```python
from build123d import *

# Parameters (mm, degrees)
MAINBODYS_W                = 20
MAINBODYS_H                = 28
MAIN_BODY_DEPTH            = 1.6
GROUND_CUT_DEPTH           = 18.278888853
MIDCUTS_W                  = 13
MIDCUTS_H                  = 7
MID_CUT_DEPTH              = 18.278888853
TOPPOWERACCESSCUTS_W       = 11.7
TOPPOWERACCESSCUTS_H       = 6.9
TOP_POWER_ACCESS_CUT_DEPTH = 18.278888853
MC_FILLET_R                = 0.5
ALL_INNER_CUTS_FILLETS_R   = 0.2
OUTER_FILLETS_R            = 1


with BuildPart() as part:
    # MainBodyS → MAIN BODY (new body)
    with BuildSketch(Plane.XY):
        Rectangle(MAINBODYS_W, MAINBODYS_H)
    extrude(amount=-MAIN_BODY_DEPTH)

    # GroundCutS → GROUND CUT (cut, through all)
    with BuildSketch(Plane.XY):
        with BuildLine():
            Line((-2.5, -7.5), (2.5, -7.5))
            ThreePointArc((2.5, -7.5), (3, -8), (2.5, -8.5))
            Line((2.5, -8.5), (-2.5, -8.5))
            ThreePointArc((-2.5, -8.5), (-3, -8), (-2.5, -7.5))
        make_face()
    extrude(amount=-GROUND_CUT_DEPTH, mode=Mode.SUBTRACT)

    # MidCutS → MID CUT (cut, through all)
    with BuildSketch(Plane.XY):
        with Locations((0, -1)):
            Rectangle(MIDCUTS_W, MIDCUTS_H)
    extrude(amount=-MID_CUT_DEPTH, mode=Mode.SUBTRACT)

    # TopPowerAccessCutS → TOP POWER ACCESS CUT (cut, through all)
    with BuildSketch(Plane.XY):
        with Locations((0, 5.95)):
            Rectangle(TOPPOWERACCESSCUTS_W, TOPPOWERACCESSCUTS_H)
    extrude(amount=-TOP_POWER_ACCESS_CUT_DEPTH, mode=Mode.SUBTRACT)

    # MC FILLET
    mc_fillet_edges = [part.edges().sort_by_distance(p)[0] for p in [
        (5.85, 2.5, -0.8),
        (-5.85, 2.5, -0.8),
    ]]
    fillet(mc_fillet_edges, radius=MC_FILLET_R)

    # ALL INNER CUTS FILLETS
    all_inner_cuts_fillets_edges = [part.edges().sort_by_distance(p)[0] for p in [
        (-6.5, -4.5, -0.8),
        (6.5, -4.5, -0.8),
        (6.5, 2.5, -0.8),
        (-6.5, 2.5, -0.8),
        (-5.85, 9.4, -0.8),
        (5.85, 9.4, -0.8),
    ]]
    fillet(all_inner_cuts_fillets_edges, radius=ALL_INNER_CUTS_FILLETS_R)

    # OUTER FILLETS
    outer_fillets_edges = [part.edges().sort_by_distance(p)[0] for p in [
        (10, -14, -0.8),
        (-10, -14, -0.8),
        (-10, 14, -0.8),
        (10, 14, -0.8),
    ]]
    fillet(outer_fillets_edges, radius=OUTER_FILLETS_R)


solid = part.part
```
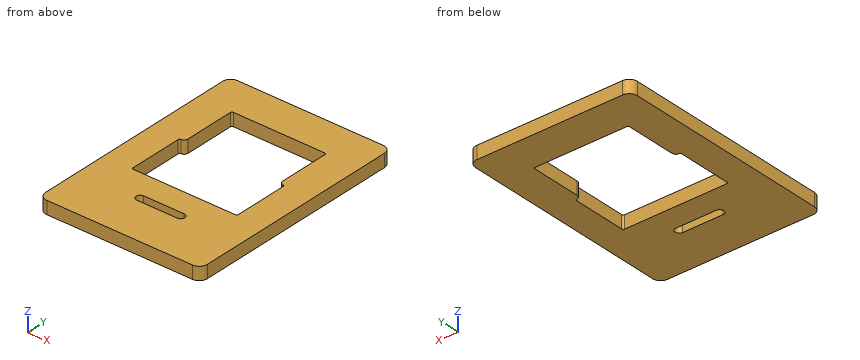
CAD build for the part. Positions are in the model's coordinates, mm. Coordinates: 2 decimals unless noted, no trailing zeros. Write each loop counter-clockwise with the first axis right and the second up, starting at its lowest first coordinate (ties: lowest second). Pieces come first, ordered by that corner, then holes. Notation, with made-up numbers: (24.25, -40) -> (40.25, -40) arc R5 ccw to (40.25, -35) -> close; hole circle Ø2 at (22.5, 35.5). An arc over 180 degrees is marked (long way). Use CSV: the item, a comma, the result in double quotes. Start each with the question number.
Item 1: Band-saw the part on A-A, the plane y = -8. Write the cut outline in (x, z), plus the area to 3 significant figures.
Item 2: Wall check: probe 1 along Y at (x, z) = (2, -1.45); probe 2 along Y at (x, z) = (-5, -1.15); probe 3 along X at (y, z) = (1.25, -1.3). Give the ranges that are in metal, low to high.
Item 3: Drop a flat-ended pin along its axis: P1, Ø12, axis at x = -2, y = 11, coming from the +Z side. Give the stop position or say it passes through.
Item 4: Band-saw the part on B-B, the plane x = -0.5. Write the cut outline in (y, z), plus the area to 3 significant figures.
Item 5: Band-saw the part on D-D, the plane y = 4. Write the cut outline in (x, z), plus the area to 3 significant figures.
Item 6: Band-saw the part on C-C, the plane z = -0.6. Give the number of separate pieces and of enclosed holes in the cut face, plus the area to 3 significant figures.
Response values:
1,outline,"(-10, -1.6) -> (-3, -1.6) -> (-3, 0) -> (-10, 0) -> close; (3, -1.6) -> (10, -1.6) -> (10, 0) -> (3, 0) -> close"
1,area,"22.4 mm2"
2,probe 1,"y = -14 to -8.5, -7.5 to -4.5, 9.4 to 14"
2,probe 2,"y = -14 to -4.5, 9.4 to 14"
2,probe 3,"x = -10 to -6.5, 6.5 to 10"
3,P1,"stops at z = 0"
4,outline,"(-14, -1.6) -> (-8.5, -1.6) -> (-8.5, 0) -> (-14, 0) -> close; (-7.5, -1.6) -> (-4.5, -1.6) -> (-4.5, 0) -> (-7.5, 0) -> close; (9.4, -1.6) -> (14, -1.6) -> (14, 0) -> (9.4, 0) -> close"
4,area,"21.0 mm2"
5,outline,"(-10, -1.6) -> (-5.85, -1.6) -> (-5.85, 0) -> (-10, 0) -> close; (5.85, -1.6) -> (10, -1.6) -> (10, 0) -> (5.85, 0) -> close"
5,area,"13.3 mm2"
6,separate pieces,"1"
6,enclosed holes,"2"
6,area,"382 mm2"
